```python
from build123d import *

# Parameters (mm, degrees)
F0_W = 3.302
F0_H = 12.7
F2_R = 5.08
F3_R = 1.27


with BuildPart() as f1:
    # F0 (on Front) → F1 (revolve)
    with BuildSketch(Plane.XZ):
        Polygon((-3.302, 0), (-17.766322, 0), (0, -38.1), (0, 0), align=None)
        with Locations((-1.651, 6.35)):
            Rectangle(F0_W, F0_H)
    revolve(axis=Axis((0, 0, -19.05), (0, 0, -1)))

    # F2
    f2_edges = [f1.edges().sort_by_distance(p)[0] for p in [
        (17.766322, 0, 0),
    ]]
    fillet(f2_edges, radius=F2_R)

    # F3
    f3_edges = [f1.edges().sort_by_distance(p)[0] for p in [
        (3.302, 0, 12.7),
    ]]
    fillet(f3_edges, radius=F3_R)


solid = f1.part
```
Design review of the part built by this model. Coordinates are the model's own, in mm. A direction names the side the tool comes from. Round coordinates to 2 decimals unless told otherwise and drop trailing zeros. Write each loop counter-clockwise with the first axis right and the second up, starting at its lowest first coordinate (ties: lowest second). Pieces come first, ordered by that corner, then holes.
Item 1: We need section A-A on z = 5. Write out the cut boundary in (x, y).
Item 2: Clearance check with flat-ended pins moving along their axes: pin 1 Ø6 at (x, z) = (3, -19.5) entering from +Y; pin 2 Ø1.5 at (x, z) = (6, -24.5) entering from -Y; pin 3 Ø10 at (y, z) = (-2, -28) entering from +X. State where each tip first meets the part, or that it passes through.
Item 3: We need section B-B on z = -22. Write out the cut boundary in (x, y), and give its area (3 significant figures).
Item 4: For faces 1 (the cylindrical face through (-3.05, -1.26, 5.8)), 2 (the conical face through (4.36, -3.35, -26.31)), list the 3-axis set-ups (+Z, -Z, +X, -X, +Y, -Y) from which the entire face can be reached by the end or side of a thin tool; tool diameter is ignored.
Item 5: For probe 1 along Z at (x, y) = (8, -6.5); probe 2 along Z at (x, y) = (2, 2.25); probe 3 along X at (y, z) = (-7, -11), list the stretches that pass through material, from the lowest coordinate up.
Returned:
1. outline: circle Ø6.6 at (0, 0)
2. pin 1: stops at y = 9.79
2. pin 2: stops at y = -3.72
2. pin 3: stops at x = 6.93
3. outline: circle Ø15.02 at (0, 0)
3. area: 177 mm2
4. face 1: +Z
4. face 2: -Z
5. probe 1: z = -15.99 to -0.03
5. probe 2: z = -31.64 to 12.24
5. probe 3: x = -10.52 to 10.52
